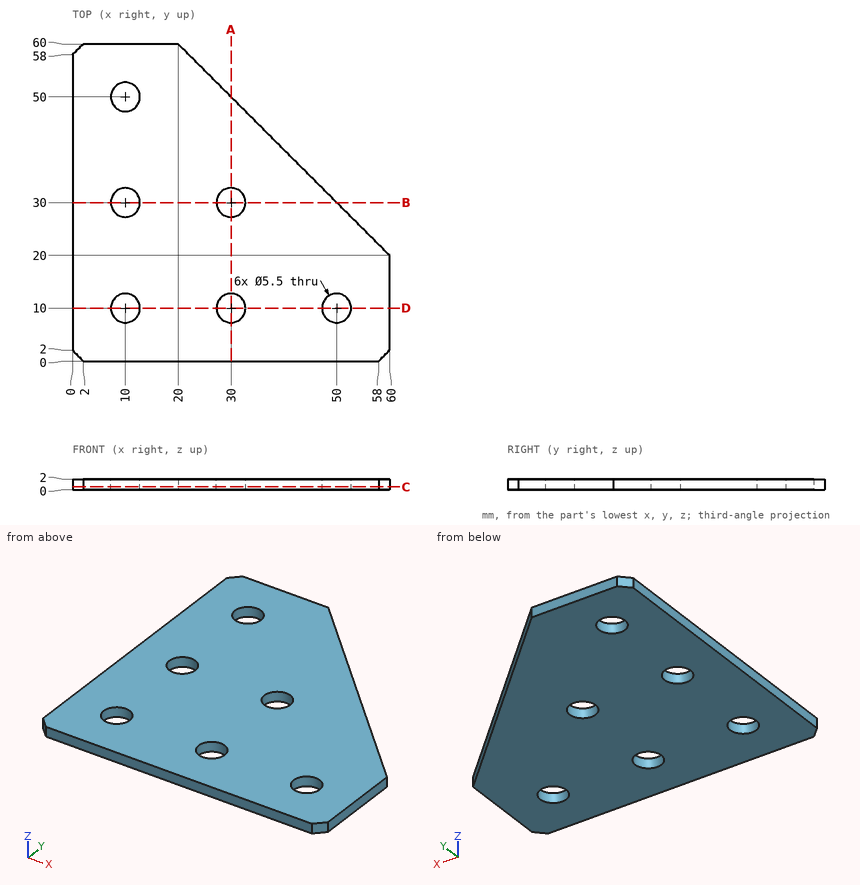
Answer from the drawing. Dimensions are ordinates in mm from the lowest x, y and z of the part. Coordinates: 2 decimals unless noted, no trailing zeros. Write each loop counter-clockwise with the first axis right and the second up, starting at its lowest first coordinate (ties: lowest second). Pieces come first, ordered by that corner, then holes. Notation, with made-up numbers: (20, -35) - (31, -35) arc R22 ccw to (31, -14) - close; hole circle Ø11 at (51, 38). An arc over 180 degrees is marked (long way). Return JSON: item names as keys, results as strings. Group by question number.
Q1. The part is cut by section A-A on x = 30. Write down the section's boundary in (y, z), and give its area (3 significant figures).
Q2. Flat-ended cylindrical pins translate along their axes: pin 1 Ø6.5 at (x, y) = (10, 50) entering from +Z; pin 2 Ø1 at (x, y) = (30, 11) entering from +Z. Find the tip coordinate at first contact, or state that the pin passes through.
Q3. The part is cut by section D-D on y = 10. Write down the section's boundary in (x, z), and give its area (3 significant figures).
Q4. Find the intervals of material crossed by line 1 along Y through (x, z) = (10, 1.65); line 2 along X through (y, z) = (30, 1.05), in increasing order. Write a range as [from, to].
Q5. The part is cut by section C-C on z = 0.5. Write down the section's boundary in (x, y).
Evaluation:
{
 "1": {"outline": "(0, 0) - (7.25, 0) - (7.25, 2) - (0, 2) - close; (12.75, 0) - (27.25, 0) - (27.25, 2) - (12.75, 2) - close; (32.75, 0) - (50, 0) - (50, 2) - (32.75, 2) - close", "area": "78.0 mm2"},
 "2": {"pin 1": "stops at z = 2", "pin 2": "passes through"},
 "3": {"outline": "(0, 0) - (7.25, 0) - (7.25, 2) - (0, 2) - close; (12.75, 0) - (27.25, 0) - (27.25, 2) - (12.75, 2) - close; (32.75, 0) - (47.25, 0) - (47.25, 2) - (32.75, 2) - close; (52.75, 0) - (60, 0) - (60, 2) - (52.75, 2) - close", "area": "87.0 mm2"},
 "4": {"line 1": "y = [0, 7.25], [12.75, 27.25], [32.75, 47.25], [52.75, 60]", "line 2": "x = [0, 7.25], [12.75, 27.25], [32.75, 50]"},
 "5": {"outline": "(0, 2) - (2, 0) - (58, 0) - (60, 2) - (60, 20) - (20, 60) - (2, 60) - (0, 58) - close; hole circle Ø5.5 at (10, 10); hole circle Ø5.5 at (10, 30); hole circle Ø5.5 at (10, 50); hole circle Ø5.5 at (30, 10); hole circle Ø5.5 at (30, 30); hole circle Ø5.5 at (50, 10)"}
}
